from build123d import *

# Parameters (mm, degrees)
BOSS_EXTRUDE1_DEPTH       = 10
SKETCH8_R                 = 5
CUT_EXTRUDE1_DEPTH        = 44.233266529
FILLET1_R                 = 30
M6X1_0_TAPPED_HOLE1_D     = 5
M6X1_0_TAPPED_HOLE2_D     = 5
M6X1_0_TAPPED_HOLE3_D     = 5
M3_CLEARANCE_HOLE2_D      = 3.5
M3_CLEARANCE_HOLE2_DEPTH  = 12.1
M3_CLEARANCE_HOLE2_TIP    = 1.051506083
F_3_0MM_DOWEL_HOLE2_D     = 3
F_3_0MM_DOWEL_HOLE2_DEPTH = 12.1
F_3_0MM_DOWEL_HOLE2_TIP   = 0.901290929
SKETCH29_R                = 10.5
CUT_EXTRUDE2_DEPTH        = 5
CHAMFER2_SIZE             = 0.5


with BuildPart() as part:
    # Sketch2 → Boss-Extrude1 (new body)
    with BuildSketch(Plane(origin=(0, 0, 0), x_dir=(1, 0, 0), z_dir=(0, 1, 0))):
        Polygon((-22.480762114, 21.062177826), (-29.480762114, 8.937822174), (-7, -4.041451884), (-7, -30), (7, -30), (7, -4.041451884), (29.480762114, 8.937822174), (22.480762114, 21.062177826), (0, 8.082903769), align=None)
    extrude(amount=BOSS_EXTRUDE1_DEPTH)

    # Sketch8 → Cut-Extrude1 (cut, through all)
    with BuildSketch(Plane(origin=(0, 10, 0), x_dir=(1, 0, 0), z_dir=(0, 1, 0))):
        with Locations(Location((0, 0, 0), (0, 0, 270))):
            Circle(SKETCH8_R)
    extrude(amount=-CUT_EXTRUDE1_DEPTH, mode=Mode.SUBTRACT)

    # Fillet1
    fillet1_edges = [part.edges().sort_by_distance(p)[0] for p in [
        (-7, 5, 4.041451884),
        (0, 5, -8.082903769),
        (7, 5, 4.041451884),
    ]]
    fillet(fillet1_edges, radius=FILLET1_R)

    # M6x1.0 Tapped Hole1 (through all)
    with Locations(Plane(origin=(-3.5, 0, -6.062177826), x_dir=(-0.8660254037844384, 0, 0.5000000000000007), z_dir=(-0.5000000000000007, 0, -0.8660254037844384))):
        with Locations((-25.68097998, 5)):
            Hole(M6X1_0_TAPPED_HOLE1_D / 2)

    # M6x1.0 Tapped Hole2 (through all)
    with Locations(Plane(origin=(3.5, 0, -6.062177826), x_dir=(-0.8660254037844383, 0, -0.5000000000000009), z_dir=(0.5000000000000008, 0, -0.8660254037844382))):
        with Locations((25.68097998, 5)):
            Hole(M6X1_0_TAPPED_HOLE2_D / 2)

    # M6x1.0 Tapped Hole3 (through all)
    with Locations(Plane(origin=(7, 0, 0), x_dir=(0, 0, -1), z_dir=(1, 0, 0))):
        with Locations((-25.68097998, 5)):
            Hole(M6X1_0_TAPPED_HOLE3_D / 2)

    # M3 Clearance Hole2
    with Locations(Plane(origin=(0, 10, 0), x_dir=(1, 0, 0), z_dir=(0, 1, 0))):
        with Locations((5.833630945, 5.833630945), (5.833630945, -5.833630945), (-5.833630945, -5.833630945), (-5.833630945, 5.833630945), (0, 0)):
            Hole(M3_CLEARANCE_HOLE2_D / 2, depth=M3_CLEARANCE_HOLE2_DEPTH)
            with Locations((0, 0, -(M3_CLEARANCE_HOLE2_DEPTH + M3_CLEARANCE_HOLE2_TIP / 2))):  # 118° drill point
                Cone(0, M3_CLEARANCE_HOLE2_D / 2, M3_CLEARANCE_HOLE2_TIP, mode=Mode.SUBTRACT)

    # Ø3.0mm Dowel Hole2
    with Locations(Plane(origin=(0, 10, 0), x_dir=(1, 0, 0), z_dir=(0, 1, 0))):
        with Locations((0, -8.25)):
            Hole(F_3_0MM_DOWEL_HOLE2_D / 2, depth=F_3_0MM_DOWEL_HOLE2_DEPTH)
            with Locations((0, 0, -(F_3_0MM_DOWEL_HOLE2_DEPTH + F_3_0MM_DOWEL_HOLE2_TIP / 2))):  # 118° drill point
                Cone(0, F_3_0MM_DOWEL_HOLE2_D / 2, F_3_0MM_DOWEL_HOLE2_TIP, mode=Mode.SUBTRACT)

    # Sketch29 → Cut-Extrude2 (cut)
    with BuildSketch(Plane(origin=(0, 10, 0), x_dir=(1, 0, 0), z_dir=(0, 1, 0))):
        with Locations(Location((0, 0, 0), (0, 0, 270))):
            Circle(SKETCH29_R)
    extrude(amount=-CUT_EXTRUDE2_DEPTH, mode=Mode.SUBTRACT)

    # Chamfer2
    chamfer2_edges = [part.edges().sort_by_distance(p)[0] for p in [
        (7, 10, 25.68097998),
        (25.980762114, 0, -15),
        (7, 0, 25.68097998),
        (0, 10, -10.5),
        (0, 0, 30),
        (-29.480762114, 5, -8.937822174),
        (-22.480762114, 5, -21.062177826),
        (22.480762114, 5, -21.062177826),
        (29.480762114, 5, -8.937822174),
        (7, 5, 30),
        (-7, 5, 30),
        (25.980762114, 10, -15),
        (18.740381057, 10, -18.902667816),
        (-25.980762114, 10, -15),
        (-25.740381057, 10, -6.778312164),
        (25.740381057, 0, -6.778312164),
        (25.740381057, 10, -6.778312164),
        (-7, 0, 25.68097998),
        (-7, 10, 25.68097998),
        (-18.740381057, 0, -18.902667816),
        (-18.740381057, 10, -18.902667816),
        (11.019237886, 0, 6.36195996),
        (11.019237886, 10, 6.36195996),
        (-11.019237886, 0, 6.36195996),
        (-11.019237886, 10, 6.36195996),
        (0, 0, -12.72391992),
        (0, 10, -12.72391992),
        (0, 10, 30),
        (-25.740381057, 0, -6.778312164),
        (-25.980762114, 0, -15),
        (18.740381057, 0, -18.902667816),
    ]]
    chamfer(chamfer2_edges, length=CHAMFER2_SIZE)


solid = part.part
CAD build for the part. Positions are in the model's coordinates, mm. A direction names the side the tool comes from. Give positions to 0.01 mm unless a question says otherwise; leave off trailing zeros. Loops run counter-clockwise (first coordinate to the right, second up) from the corner with the lowest first, then second, coordinate; pieces in that order, holes last. Notation, with made-up numbers: M 64,80.5 L 77,80.5 A27 cw 77,109.5 Z; hole C 44,10.5 d8. An arc over 180 degrees is marked long. Answer in a Markdown table with one row per item. Add a question column.
Item 1: Drop flat-ended pins along their axis: P1, Ø17, axis at x = 0, z = 0, coming from the +Y side; P2, Ø5, axis at x = 12, y = 4, coming from the +Z side; P3, Ø4, axis at y = 5, z = 26.5, coming from the -X side. Give the stop position or say it passes through.
Item 2: Probe probe 1 along Z at (x, y) = (1, 7.25); probe 2 along Z at (x, y) = (6, 3); probe 3 along Y at (x, z) = (21, -17.5). List the from-to ranges inside material, lowest first.
Item 3: Band-saw the part on B-B on x = 0. Give the cut face in (y, z).
Item 4: Band-saw the part on D-D on y = 1.75. Give the cut face in (x, z).
Item 5: Band-saw the part on A-A on y = 6.25. Give the number of separate pieces and of enclosed holes in the cut face, then the cut area to 3 significant figures.
Item 6: Mould opens along Y. For faces 4 (the face through (-21.1, 7.1, -12.1)), 5 (the face through (18.7, 9.75, -18.59)), 6 (the face through (-18.6, 0.25, -18.53)), 7 (the face through (-0.22, 5.063, -12.725)) say: +Y half, -Y half, draft (parallel to the pull), parting line (faces both ways), or undercut.
Item 7: Band-saw the part on C-C on z = 27. Give the cut face in (x, y), then the cut area to 3 significant figures.
Item 8: Tool access for faces 1 (the face through (0, 5, 30)), 2 (the face through (3.2, 7.3, 10)), 3 (the face through (17, 6.9, -17.9)): list every direction of +Z, -Z, +X, -X, +Y, -Y with a clear straight run to the whole face (end or side of a thin tool).
Reply:
| question | item | result |
|---|---|---|
| 1 | P1 | stops at y = 5 |
| 1 | P2 | stops at z = 9.37 |
| 1 | P3 | stops at x = -7 |
| 2 | probe 1 | z = -12.74 to -10.45, 10.45 to 24.59, 26.77 to 30 |
| 2 | probe 2 | z = -13.33 to -7.58, -4.09 to 4.09, 7.58 to 24.18, 27.18 to 30 |
| 2 | probe 3 | y = 0 to 2.84, 7.16 to 10 |
| 3 | outline | M 0,-12.22 L 0.5,-12.72 L 9.5,-12.72 L 10,-12.22 L 10,-11 L 9.5,-10.5 L 5,-10.5 L 5,-5 L 0,-5 Z; M 0,5 L 5,5 L 5,6.75 L 0,6.75 Z; M 0,9.75 L 5,9.75 L 5,10.5 L 9.5,10.5 L 10,11 L 10,29.5 L 9.5,30 L 0.5,30 L 0,29.5 Z; hole C 5,25.68 d5 |
| 4 | outline | M -29.23,-9.37 L -22.73,-20.63 L -22.05,-20.81 L -15,-16.74 A30 cw 15,-16.74 L 22.05,-20.81 L 22.73,-20.63 L 29.23,-9.37 L 29.05,-8.69 L 22,-4.62 A30 cw 7,21.36 L 7,29.5 L 6.5,30 L -6.5,30 L -7,29.5 L -7,21.36 A30 cw -22,-4.62 L -29.05,-8.69 Z; hole C -5.83,-5.83 d3.5; hole C -5.83,5.83 d3.5; hole C 0,0 d10; hole C 0,8.25 d3; hole C 5.83,-5.83 d3.5; hole C 5.83,5.83 d3.5 |
| 5 | separate pieces | 4 |
| 5 | enclosed holes | 1 |
| 5 | area | 791 mm^2 |
| 6 | face 4 | undercut |
| 6 | face 5 | +Y half |
| 6 | face 6 | -Y half |
| 6 | face 7 | draft |
| 7 | outline | M -7,0.5 L -6.5,0 L 6.5,0 L 7,0.5 L 7,2.88 L -7,2.88 Z; M -7,7.12 L 7,7.12 L 7,9.5 L 6.5,10 L -6.5,10 L -7,9.5 Z |
| 7 | area | 80.0 mm^2 |
| 8 | face 1 | +Z, +X, -X, +Y, -Y |
| 8 | face 2 | +Y |
| 8 | face 3 | -Z, +Y, -Y |
